Verification items for the finished model (mm, model axes). Face numbers are marked on the shaded views. A direction names the side the tool comes from. Round coordinates to 2 decimals unless told otherwise and drop trailing zeros. Order: outer loops, then holes, each group sorted by start corner. A loop starts at its lowest first (then second) coordinate and runs counter-clockwise, first axis right, second up. Notation, with made-up numbers: (11.25, 38.5) -> (45.25, 38.5) arc R24 cw to (45.25, 69.5) -> close; hole circle Ø9 at (6.5, -33). An arc over 180 degrees is marked (long way). Put each result on its own line as item: value.
```python
from build123d import *

# Parameters (mm, degrees)
EXTRUDE_3_DEPTH     = 80
CUT_EXTRUDE_1_DEPTH = 78


with BuildPart() as part:
    # 草图1 → 凸台-拉伸3 (new body)
    with BuildSketch(Plane(origin=(0, 0, 0), x_dir=(1, 0, 0), z_dir=(0, 1, 0))):
        Polygon((-1.656854249, 4), (69.656854249, 4), (128.568542495, -54.911688245), (128.568542495, -160.225396744), (69.656854249, -219.13708499), (-1.656854249, -219.13708499), (-60.568542495, -160.225396744), (-60.568542495, -54.911688245), align=None)
    extrude(amount=EXTRUDE_3_DEPTH)

    # 草图1<6> → 切除-拉伸1 (cut)
    with BuildSketch(Plane(origin=(0, 0, 0), x_dir=(1, 0, 0), z_dir=(0, 1, 0))):
        Polygon((-58.568542495, -55.74011537), (-0.828427125, 2), (68.828427125, 2), (126.568542495, -55.74011537), (126.568542495, -159.39696962), (68.828427125, -217.13708499), (-0.828427125, -217.13708499), (-58.568542495, -159.39696962), align=None)
    extrude(amount=CUT_EXTRUDE_1_DEPTH, mode=Mode.SUBTRACT)


solid = part.part
```
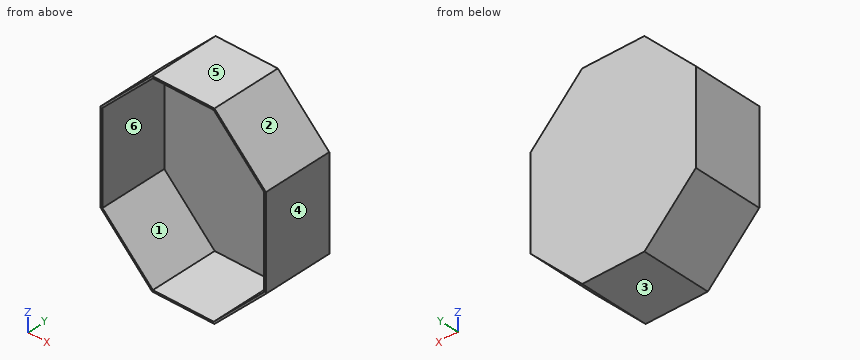
Item 1: Sectioned sample at B-B, the plane x = 36. Record the boundary of the cut face in (y, z).
Geometry check:
outline: (0, -4) -> (80, -4) -> (80, 219.14) -> (0, 219.14) -> (0, 217.14) -> (78, 217.14) -> (78, -2) -> (0, -2) -> close
Item 2: Release check for a two-part mould opening along Z. For the marked faces 1, 2, 3 and 4 record: pulls with the +Z half, pulls with the -Z half, needs draft (parallel to the pull), parting line crosses it, or undercut.
Geometry check:
face 1: undercut
face 2: pulls with the +Z half
face 3: pulls with the -Z half
face 4: needs draft
Item 3: Material ranges on line 1 along X through (y, z) = (56, 85.5); line 2 along Z through (x, y) = (10, 43.5); line 3 along Y through (x, z) = (41.5, 142), recorded low to high.
Geometry check:
line 1: -60.57 to -58.57, 126.57 to 128.57
line 2: -4 to -2, 217.14 to 219.14
line 3: 78 to 80
Item 4: Sectioned sample at C-C, the plane z = 96. Record the boundary of the cut face in (x, y), then the cut area to 3 significant figures.
Geometry check:
outline: (-60.57, 0) -> (-58.57, 0) -> (-58.57, 78) -> (126.57, 78) -> (126.57, 0) -> (128.57, 0) -> (128.57, 80) -> (-60.57, 80) -> close
area: 690 mm2
Item 5: Tool access check on the marked faces 5 and 6. Record the directions out of +Z, -Z, +X, -X, +Y, -Y that give a thin tool (end or side, any length) a straight path to the whole face; none if there is none.
Geometry check:
face 5: +Z, +X, -X, +Y, -Y
face 6: -Y
Item 6: Sectioned sample at A-A, the plane y = 32.5. Record the boundary of the cut face in (x, z), then the cut area to 3 significant figures.
Geometry check:
outline: (-60.57, 54.91) -> (-1.66, -4) -> (69.66, -4) -> (128.57, 54.91) -> (128.57, 160.23) -> (69.66, 219.14) -> (-1.66, 219.14) -> (-60.57, 160.23) -> close; hole (-58.57, 55.74) -> (-0.83, -2) -> (68.83, -2) -> (126.57, 55.74) -> (126.57, 159.4) -> (68.83, 217.14) -> (-0.83, 217.14) -> (-58.57, 159.4) -> close
area: 1,360 mm2
Item 7: Depth check by flat-ended pin: pin 1 Ø8 at (y, z) = (22, 43) entering from -X; pin 2 Ø6 at (x, z) = (94, 95) entering from -Y; pin 3 Ø10 at (y, z) = (30.5, 181.5) entering from +X. Enter the tip coordinate at first touch or a pass-through.
Geometry check:
pin 1: x = -52.66
pin 2: y = 78
pin 3: x = 112.29
